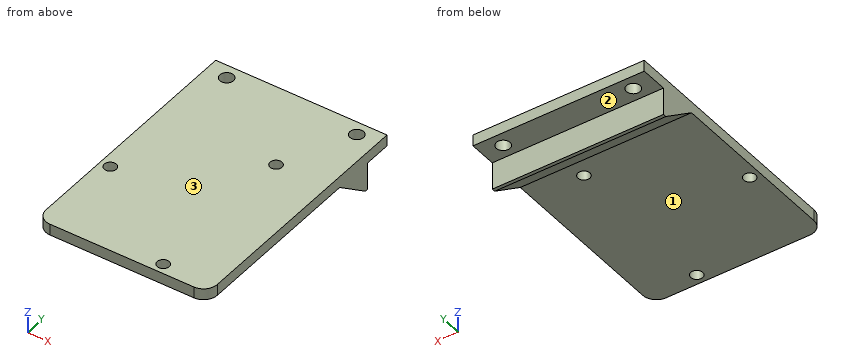
from build123d import *

# Parameters (mm, degrees)
SKETCH_1_W      = 50
SKETCH_1_H      = 74.4
SKETCH_1_R      = 1.75
SKETCH_1_R_2    = 2
EXTRUDE_2_DEPTH = 3.3
FILLET_1_R      = 4
EXTRUDE_3_DEPTH = 50


with BuildPart() as part:
    # ｽｹｯﾁ1 → ﾎﾞｽ - 押し出し2 (new body)
    with BuildSketch(Plane.XY):
        with Locations((-9.92, -12.6)):
            Rectangle(SKETCH_1_W, SKETCH_1_H)
        Circle(SKETCH_1_R, mode=Mode.SUBTRACT)
        with Locations((0, -46.8)):
            Circle(SKETCH_1_R, mode=Mode.SUBTRACT)
        with Locations((-31.92, -23.4)):
            Circle(SKETCH_1_R, mode=Mode.SUBTRACT)
        with Locations((9.08, 20.6)):
            Circle(SKETCH_1_R_2, mode=Mode.SUBTRACT)
        with Locations((-28.92, 20.6)):
            Circle(SKETCH_1_R_2, mode=Mode.SUBTRACT)
    extrude(amount=EXTRUDE_2_DEPTH)

    # ﾌｨﾚｯﾄ1
    fillet_1_edges = [part.edges().sort_by_distance(p)[0] for p in [
        (15.08, -49.8, 1.65),
        (-34.92, -49.8, 1.65),
    ]]
    fillet(fillet_1_edges, radius=FILLET_1_R)

    # ｽｹｯﾁ3 → ﾎﾞｽ - 押し出し3 (add)
    with BuildSketch(Plane(origin=(15.08, 0, 0), x_dir=(0, 0, -1), z_dir=(1, 0, 0))):
        Polygon((0, 16.6), (8, 16.6), (8, 15.6), (0, 5), align=None)
    extrude(amount=-EXTRUDE_3_DEPTH)


solid = part.part
The model under review builds one solid part; all positions refer to its coordinate system, in mm. Face numbers are marked on the shaded views. A direction names the side the tool comes from. Round coordinates to 2 decimals unless told otherwise and drop trailing zeros. Write each loop counter-clockwise with the first axis right and the second up, starting at its lowest first coordinate (ties: lowest second). Pieces come first, ordered by that corner, then holes. Notation, with made-up numbers: M 46.25,83.5 L 104.25,83.5 A16 ccw 104.25,105.5 Z; hole C 44.5,57 d10. An arc over 180 degrees is marked long. Use a Markdown table: item, result. Add a question column.
Q1. We need section B-B, the plane x = -28.92. State the section outline as (y, z) points, plus the area to 3 significant figures.
Q2. We need section D-D, the plane x = -1. State the section outline as (y, z) points.
Q3. To check wall thickness, follow line 1 (Y direction, x = -28.92, z = 2.2); line 2 (Z direction, x = -32, y = -8); line 3 (Y direction, x = -3.5, z = -4.5). State the ranges of each line that lie inside material, in increasing order.
Q4. We need section C-C, the plane y = 0. State the section outline as (x, z) points, plus the area to 3 significant figures.
Q5. We need section A-A, the plane y = 20.6. State the section outline as (x, z) points.
Q6. Machinability: for the marked faces 1, 2 and 3, which of the approach directions +Z, -Z, +X, -X, +Y, -Y give a long, thin tool a straight path to every point of the face, cutting with its end or side? Answer none if there is none.
Q7. Insertion check: pin 1 (15 mm diameter, centred on x = 0, y = -17.5, fed in from -Z); pin 2 (6 mm diameter, centred on x = -21.5, z = -4, fed in from -Y) (3 decimals); pin 3 (2.5 mm diameter, centred on x = -10.5, z = -3.5, fed in from +Y); pin 4 (3 mm diameter, centred on x = -31.92, y = -23.4, fed in from -Z). Each pin has a flat end and moves straight along its axis. Give the tip position at first contact, or say it passes through.
Findings below:
| question | item | result |
|---|---|---|
| 1 | outline | M -49.8,0 L 5,0 L 15.6,-8 L 16.6,-8 L 16.6,0 L 18.6,0 L 18.6,3.3 L -49.8,3.3 Z; M 22.6,0 L 24.6,0 L 24.6,3.3 L 22.6,3.3 Z |
| 1 | area | 283 mm² |
| 2 | outline | M -49.8,0 L -48.24,0 L -48.24,3.3 L -49.8,3.3 Z; M -45.36,0 L -1.44,0 L -1.44,3.3 L -45.36,3.3 Z; M 1.44,0 L 5,0 L 15.6,-8 L 16.6,-8 L 16.6,0 L 24.6,0 L 24.6,3.3 L 1.44,3.3 Z |
| 3 | line 1 | y = -49.8 to 18.6, 22.6 to 24.6 |
| 3 | line 2 | z = 0 to 3.3 |
| 3 | line 3 | y = 10.96 to 16.6 |
| 4 | outline | M -34.92,0 L -1.75,0 L -1.75,3.3 L -34.92,3.3 Z; M 1.75,0 L 15.08,0 L 15.08,3.3 L 1.75,3.3 Z |
| 4 | area | 153 mm² |
| 5 | outline | M -34.92,0 L -30.92,0 L -30.92,3.3 L -34.92,3.3 Z; M -26.92,0 L 7.08,0 L 7.08,3.3 L -26.92,3.3 Z; M 11.08,0 L 15.08,0 L 15.08,3.3 L 11.08,3.3 Z |
| 6 | face 1 | -Z, +X, -X, -Y |
| 6 | face 2 | -Z, +X, -X, +Y |
| 6 | face 3 | +Z, +X, -X, +Y, -Y |
| 7 | pin 1 | stops at z = 0 |
| 7 | pin 2 | stops at y = 6.325 |
| 7 | pin 3 | stops at y = 16.6 |
| 7 | pin 4 | passes through |
